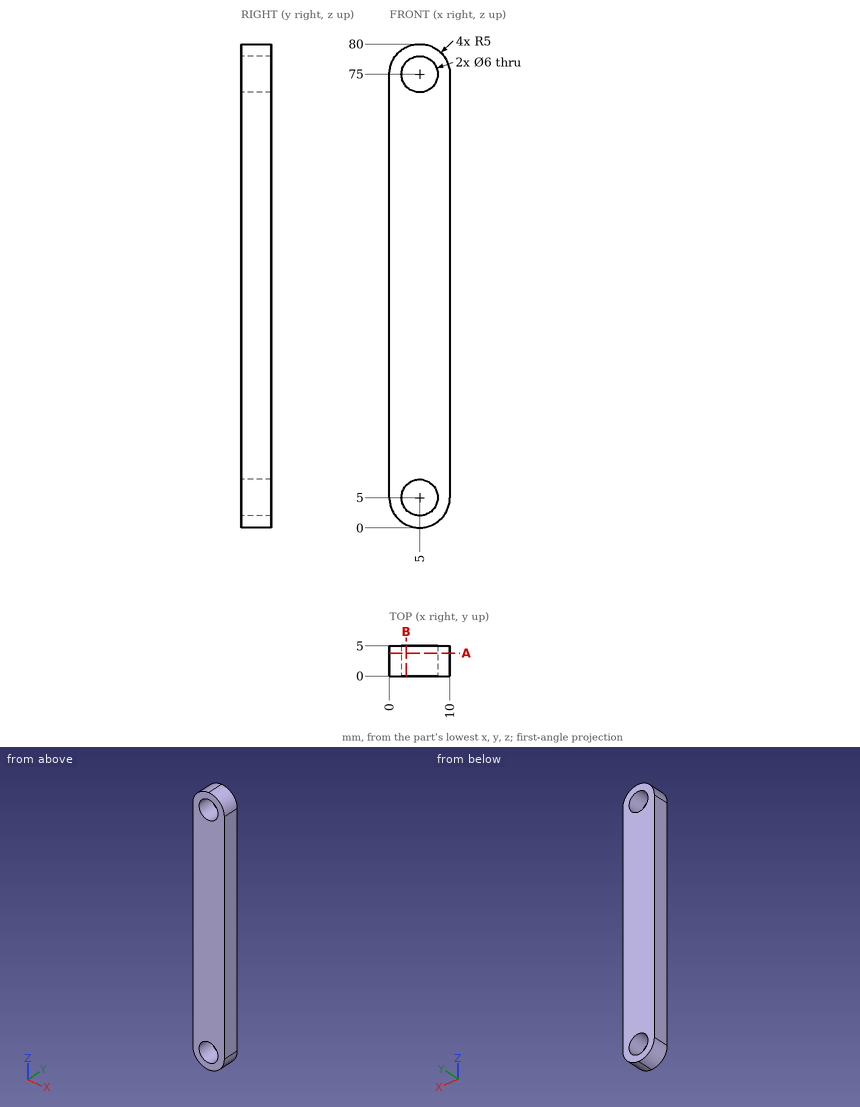
Print and shaded views of the part. All mm, measured from the part's lowest x, y and z. Round coordinates to 2 decimals unless told otherwise and drop trailing zeros. Loops run counter-clockwise (first coordinate to the right, second up) from the corner with the lowest first, then second, coordinate; pieces in that order, holes last. Notation, with made-up numbers: (12, -1.75) -> (29, -1.75) arc R32 ccw to (29, 27.25) -> close; hole circle Ø9 at (17.25, -13). An arc over 180 degrees is marked (long way). Use CSV: the item, a comma, the result in double quotes. Start each with the question number.
1) Cut at A-A, the plane y = 3.8. Give the number of separate pieces and of enclosed holes in the cut face, plus the area to 3 significant figures.
2) Wall check: L1, parallel to Z at x = 4.75, y = 3.3; L2, parallel to Z at x = 6.75, y = 4; L3, parallel to X at y = 1.05, z = 6.5. Give the ranges that are in metal, low to high. Write a range as [from, to].
3) Cut at B-B, the plane x = 2.75. Write the cut outline in (y, z) (1 decimal), plus the area to 3 significant figures.
4) Drop flat-ended pins along their axis: P1, Ø3, axis at x = 8.5, y = 3, coming from the +Z side; P2, Ø2, axis at x = 2, y = 4.5, coming from the -Z side; P3, Ø3, axis at x = 1.5, z = 69, coming from the -Y side. Give the stop position or say it passes through.
Determined:
1,separate pieces,"1"
1,enclosed holes,"2"
1,area,"722 mm2"
2,L1,"z = [0.01, 2.01], [7.99, 72.01], [77.99, 79.99]"
2,L2,"z = [0.32, 2.56], [7.44, 72.56], [77.44, 79.68]"
2,L3,"x = [0, 2.4], [7.6, 10]"
3,outline,"(0, 0.5) -> (5, 0.5) -> (5, 3) -> (0, 3) -> close; (0, 7) -> (5, 7) -> (5, 73) -> (0, 73) -> close; (0, 77) -> (5, 77) -> (5, 79.5) -> (0, 79.5) -> close"
3,area,"355 mm2"
4,P1,"stops at z = 79.58"
4,P2,"stops at z = 0.42"
4,P3,"stops at y = 0"
